Build history of the part. All positions in model axes, mm. Round coordinates to 2 decimals unless told otherwise and drop trailing zeros. Loops run counter-clockwise (first coordinate to the right, second up) from the corner with the lowest first, then second, coordinate; pieces in that order, holes last. Notation, with made-up numbers: M 4.25,31 L 18.25,31 A25 ccw 18.25,48 Z; hole C -14,-8 d10. An arc over 180 degrees is marked long. One line per item, written item: value.
```python
from build123d import *

# Parameters (mm, degrees)
ESQUISSE1_R        = 1.5
BOSS_EXTRU_2_DEPTH = 3


with BuildPart() as part:
    # Esquisse1 → Boss.-Extru.2 (new body)
    with BuildSketch(Plane.XY):
        with BuildLine():
            ThreePointArc((-2.411034891, 11.820685714), (0, 10.75), (2.411034891, 11.820685714))
            ThreePointArc((2.411034891, 11.820685714), (3.975330286, 12.779130538), (5.80943088, 12.737759334))
            ThreePointArc((5.80943088, 12.737759334), (11.865562564, 7.430237213), (13.995977593, -0.335575935))
            ThreePointArc((13.995977593, -0.335575935), (13.382779595, -2.564868949), (11.442531564, -3.822325392))
            ThreePointArc((11.442531564, -3.822325392), (9.309773091, -5.375), (9.031496673, -7.998360322))
            ThreePointArc((9.031496673, -7.998360322), (9.079386541, -9.832302285), (8.126507731, -11.399994391))
            ThreePointArc((8.126507731, -11.399994391), (4.266150404, -13.334165168), (0, -14))
            ThreePointArc((0, -14), (-3.25, -10.75), (0, -7.5))
            ThreePointArc((0, -7.5), (6.495190528, 3.75), (-6.495190528, 3.75))
            ThreePointArc((-6.495190528, 3.75), (-10.934773091, 2.560417438), (-12.124355653, 7))
            ThreePointArc((-12.124355653, 7), (-9.780131311, 10.017436376), (-6.707371512, 12.288660114))
            ThreePointArc((-6.707371512, 12.288660114), (-4.47014813, 12.872261577), (-2.411034891, 11.820685714))
        make_face()
        with Locations((9.309773091, 5.375)):
            Circle(ESQUISSE1_R, mode=Mode.SUBTRACT)
        with Locations((0, -10.75)):
            Circle(ESQUISSE1_R, mode=Mode.SUBTRACT)
        with Locations((-9.309773091, 5.375)):
            Circle(ESQUISSE1_R, mode=Mode.SUBTRACT)
    extrude(amount=BOSS_EXTRU_2_DEPTH)


solid = part.part
```
Item 1: Slice it at D-D, the plane y = 0. Give the cut face in (x, z), and give its area (3 significant figures).
Check values:
outline: M 7.5,0 L 14,0 L 14,3 L 7.5,3 Z
area: 19.5 mm2
Item 2: Pull direction X, two halves, no side cores. Call faces 1 (the face through (-3.25, -10.82, 1.48)), 2 (the face through (6.6, 3.56, 1.48)), 3 (the face through (11.804, 7.527, 1.479)), 4 (the face through (-10.872, 2.525, 1.479)): pulls with the +X half, pulls with the -X half, needs draft (parallel to the pull), parting line crosses it, or undercut.
Check values:
face 1: pulls with the -X half
face 2: undercut
face 3: pulls with the +X half
face 4: undercut
Item 3: Slice it at B-B, the plane y = -10.75. Give the cut face in (x, z).
Check values:
outline: M -3.25,0 L -1.5,0 L -1.5,3 L -3.25,3 Z; M 1.5,0 L 8.68,0 L 8.68,3 L 1.5,3 Z
Item 4: Slice it at A-A, the plane x = -8.75. Give the cut face in (y, z), and give its area (3 significant figures).
Check values:
outline: M 2.17,0 L 3.98,0 L 3.98,3 L 2.17,3 Z; M 6.77,0 L 10.93,0 L 10.93,3 L 6.77,3 Z
area: 17.9 mm2
Item 5: Drop flat-ended pins along their axis: P1, Ø1.5, axis at x = 1, z = 2, coming from the +Y side; P2, Ø2.5, axis at x = 9.31, y = 5.38, coming from the +Z side. Give the stop position or say it passes through.
Check values:
P1: stops at y = 11.26
P2: passes through
Item 6: Slice it at C-C, the plane z = 1.5. Give the number of separate pieces and of enclosed holes in the cut face, and give its area (3 significant figures).
Check values:
separate pieces: 1
enclosed holes: 3
area: 268 mm2
Item 7: Wall check: line 1 along X through (y, z) = (0, 1); line 2 along Y through (x, z) = (3.25, 2.75); line 3 along X through (y, z) = (11, 1.15). Give the ranges that are in metal, low to high.
Check values:
line 1: x = 7.5 to 14
line 2: y = -13.62 to -6.76, 6.76 to 12.49
line 3: x = -8.66 to -1.25, 1.25 to 8.66
